The listing builds one solid part. Answer for the finished solid, in the listing's coordinates (mm). A direction names the side the tool comes from. Give positions to 0.01 mm unless a question says otherwise; leave off trailing zeros. Order: outer loops, then holes, each group sorted by start corner. A loop starts at its lowest first (then second) coordinate and runs counter-clockwise, first axis right, second up. Notation, with made-up numbers: (76.5, 82) - (91.5, 82) arc R13 cw to (91.5, 98) - close; hole circle Ø1 at (-33.5, 61). An arc over 180 degrees is marked (long way). Answer as a JSON object with one key per item and string values. Group by question number.
Q1. A cutting plane is placed at A-A, the plane z = 11.25. Give the vertices of the cut face in (x, y), and give its area (3 significant figures).
Q2. Consider line 1 (Y direction, x = -8.75, z = -9); line 2 (X direction, y = -23, z = -7). Determine where each line is inside the solid, lowest interval first.
Q3. A cutting plane is placed at D-D, the plane z = 5.5. Give the vertices of the cut face in (x, y), and give its area (3 significant figures).
Q4. The mould has two halves that part along Y. Classify faces 5 (the face through (-6.35, -3, -7)), 6 (the face through (-10, -6.35, -8)): released by +Y, released by -Y, zero draft, split by the parting line, or undercut.
Q5. A cutting plane is placed at B-B, the plane y = -7.75. Give the vertices of the cut face in (x, z) (3 decimals), and give its area (3 significant figures).
Q6. For faces 1 (the face through (-6.35, -13, -3)), 2 (the face through (6.35, -3, -7)), 3 (the face through (6.35, -22, 3)), 4 (the face through (-10, -13, 0)), determine the directions among +Z, -Z, +X, -X, +Y, -Y from which every point of the face is accessible in a straight line to the end or side of a thin tool.
Q7. Given pin 1 (7 mm diameter, centred on x = 10, y = -10.5, fed in from +Z); pin 2 (5 mm diameter, centred on x = -4, z = -3.5, fed in from +Y); pin 3 (7 mm diameter, centred on x = -2, y = -23, fed in from -Z) (3 decimals); pin 4 (1.5 mm diameter, centred on x = -1.5, y = -7.5, fed in from +Z), each flat-ended and moving along its own axis, determine where each tip first touches the part or whether it passes through.
Q8. A cutting plane is placed at C-C, the plane x = 3.5. Give the vertices of the cut face in (y, z) (3 decimals), and give its area (3 significant figures).
from build123d import *

# Parameters (mm, degrees)
F0_W     = 25.4
F0_H     = 25.4
F1_DEPTH = 25.4
F2_W     = 12.7
F2_H     = 6.985
F2_H_2   = 6.35
F3_DEPTH = 25.401
F4_W     = 12.7
F4_H     = 12.7
F5_DEPTH = 25.401
F6_W     = 12.7
F6_H     = 6.985
F7_DEPTH = 25.401
F8_W     = 12.7
F8_H     = 12.7
F9_DEPTH = 12.701
F10_SIZE = 5.08


with BuildPart() as f1:
    # F0 (on Front) → F1 (new body)
    with BuildSketch(Plane.XZ):
        Rectangle(F0_W, F0_H)
    extrude(amount=F1_DEPTH)

    # F2 (on face) → F3 (cut, through all)
    with BuildSketch(Plane.XZ.offset(25.4)):
        with Locations((0, -9.2075)):
            Rectangle(F2_W, F2_H)
        with Locations((0, 3.175)):
            Rectangle(F2_W, F2_H_2)
    extrude(amount=-F3_DEPTH, mode=Mode.SUBTRACT)

    # F4 (on face) → F5 (cut, through all)
    with BuildSketch(Plane(origin=(-12.7, 0, 0), x_dir=(0, -1, 0), z_dir=(-1, 0, 0))):
        with Locations((12.7, 6.35)):
            Rectangle(F4_W, F4_H)
    extrude(amount=-F5_DEPTH, mode=Mode.SUBTRACT)

    # F6 (on face) → F7 (cut, through all)
    with BuildSketch(Plane.YZ.offset(12.7)):
        with Locations((-12.7, -9.2075)):
            Rectangle(F6_W, F6_H)
    extrude(amount=-F7_DEPTH, mode=Mode.SUBTRACT)

    # F8 (on face) → F9 (cut, through all)
    with BuildSketch(Plane.XY):
        with Locations((0, -12.7)):
            Rectangle(F8_W, F8_H)
    extrude(amount=-F9_DEPTH, mode=Mode.SUBTRACT)

    # F10
    f10_edges = [f1.edges().sort_by_distance(p)[0] for p in [
        (6.35, -22.225, -12.7),
        (6.35, -3.175, -12.7),
        (-6.35, -3.175, -12.7),
        (-6.35, -22.225, -12.7),
        (12.7, -3.175, 12.7),
        (12.7, -22.225, 12.7),
        (-12.7, -22.225, 12.7),
        (-12.7, -3.175, 12.7),
    ]]
    chamfer(f10_edges, length=F10_SIZE)


solid = f1.part
Reply:
{
 "1": {"outline": "(-9.07, -25.4) - (9.07, -25.4) - (9.07, -19.05) - (-9.07, -19.05) - close; (-9.07, -6.35) - (9.07, -6.35) - (9.07, 0) - (-9.07, 0) - close", "area": "230 mm^2"},
 "2": {"line 1": "y = -25.4 to -19.05, -6.35 to 0", "line 2": "x = -12.7 to -6.35, 6.35 to 12.7"},
 "3": {"outline": "(-12.7, -25.4) - (-6.35, -25.4) - (-6.35, -19.05) - (-12.7, -19.05) - close; (-12.7, -6.35) - (-6.35, -6.35) - (-6.35, 0) - (-12.7, 0) - close; (6.35, -25.4) - (12.7, -25.4) - (12.7, -19.05) - (6.35, -19.05) - close; (6.35, -6.35) - (12.7, -6.35) - (12.7, 0) - (6.35, 0) - close", "area": "161 mm^2"},
 "4": {"face 5": "zero draft", "face 6": "undercut"},
 "5": {"outline": "(-12.7, -5.715) - (-6.35, -5.715) - (-6.35, 0) - (-12.7, 0) - close; (6.35, -5.715) - (12.7, -5.715) - (12.7, 0) - (6.35, 0) - close", "area": "72.6 mm^2"},
 "6": {"face 1": "+Z, -Z", "face 2": "-Z, +Y, -Y", "face 3": "+Y, -Y", "face 4": "+Z, +X, -X"},
 "7": {"pin 1": "stops at z = 0", "pin 2": "stops at y = 0", "pin 3": "stops at z = -5.715", "pin 4": "passes through"},
 "8": {"outline": "(-25.4, -5.715) - (-19.05, -5.715) - (-19.05, 0) - (-25.4, 0) - close; (-25.4, 6.35) - (-19.05, 6.35) - (-19.05, 12.7) - (-25.4, 12.7) - close; (-6.35, -5.715) - (0, -5.715) - (0, 0) - (-6.35, 0) - close; (-6.35, 6.35) - (0, 6.35) - (0, 12.7) - (-6.35, 12.7) - close", "area": "153 mm^2"}
}
